from build123d import *

# Parameters (mm, degrees)
SKETCH1_R                  = 92.5
BOSS_EXTRUDE1_DEPTH        = 12
SKETCH2_OUTSIDE_W          = 239.38
SKETCH2_OUTSIDE_H          = 239.38
SKETCH2_OUTSIDE_W_2        = 140
SKETCH2_OUTSIDE_H_2        = 140
CUT_EXTRUDE1_DEPTH         = 132.363998112
SKETCH3_R                  = 65
CUT_EXTRUDE2_DEPTH         = 100.719606899
F_12_0_12_DIAMETER_HOLE1_D = 12


with BuildPart() as part:
    # Sketch1 → Boss-Extrude1 (new body)
    with BuildSketch(Plane.XY):
        Circle(SKETCH1_R)
    extrude(amount=BOSS_EXTRUDE1_DEPTH)

    # Sketch2 outside → Cut-Extrude1 (cut, through all)
    with BuildSketch(Plane.XY.offset(12)):
        Rectangle(SKETCH2_OUTSIDE_W, SKETCH2_OUTSIDE_H)
        Rectangle(SKETCH2_OUTSIDE_W_2, SKETCH2_OUTSIDE_H_2, mode=Mode.SUBTRACT)
    extrude(amount=-CUT_EXTRUDE1_DEPTH, mode=Mode.SUBTRACT)

    # Sketch3 → Cut-Extrude2 (cut, through all)
    with BuildSketch(Plane.XY.offset(12)):
        Circle(SKETCH3_R)
    extrude(amount=-CUT_EXTRUDE2_DEPTH, mode=Mode.SUBTRACT)

    # Ø12.0 (12) Diameter Hole1 (through all)
    with Locations(Plane.XY.offset(12)):
        with Locations((56.568542495, 56.568542495), (-56.568542495, 56.568542495), (-56.568542495, -56.568542495), (56.568542495, -56.568542495)):
            Hole(F_12_0_12_DIAMETER_HOLE1_D / 2)


solid = part.part
Part model, mm, in its own coordinate system. Give positions to 0.01 mm unless a question says otherwise; leave off trailing zeros. Loops run counter-clockwise (first coordinate to the right, second up) from the corner with the lowest first, then second, coordinate; pieces in that order, holes last.
(1) Band-saw the part on A-A (x = 39). Write the cut outline in (y, z), and give its area (3 significant figures).
Return value:
outline: (-70, 0) - (-52, 0) - (-52, 12) - (-70, 12) - close; (52, 0) - (70, 0) - (70, 12) - (52, 12) - close
area: 432 mm2
(2) Pull direction X, two halves, no side cores. Call faces 1 (the cylindrical face through (65.341, -65.474, 5.916)), 2 (the flat face through (-1, 70, 6)), 3 (the cylindrical face through (-62.11, 54.27, 5.92)), 4 (the flat face through (-70, -1, 6)): pulls with the +X half, pulls with the -X half, needs draft (parallel to the pull), parting line crosses it, or undercut.
Return value:
face 1: pulls with the +X half
face 2: needs draft
face 3: undercut
face 4: pulls with the -X half
(3) Band-saw the part on B-B (y = -16). Write the cut outline in (x, z).
Return value:
outline: (-70, 0) - (-63, 0) - (-63, 12) - (-70, 12) - close; (63, 0) - (70, 0) - (70, 12) - (63, 12) - close
(4) Drill centre lines: line 1 along Y through (x, z) = (2.5, 5); line 2 along Y through (x, z) = (16.5, 2.75); line 3 along Y through (x, z) = (-56.5, 6). Where is each one in solid material? Low to high.
Return value:
line 1: y = -70 to -64.95, 64.95 to 70
line 2: y = -70 to -62.87, 62.87 to 70
line 3: y = -70 to -62.57, -50.57 to -32.14, 32.14 to 50.57, 62.57 to 70
(5) Band-saw the part on C-C (z = 6). Write the cut outline in (x, y).
Return value:
outline: (-70, -60.47) arc R92.5 ccw to (-60.47, -70) - (60.47, -70) arc R92.5 ccw to (70, -60.47) - (70, 60.47) arc R92.5 ccw to (60.47, 70) - (-60.47, 70) arc R92.5 ccw to (-70, 60.47) - close; hole circle Ø130 at (0, 0); hole circle Ø12 at (-56.57, -56.57); hole circle Ø12 at (-56.57, 56.57); hole circle Ø12 at (56.57, -56.57); hole circle Ø12 at (56.57, 56.57)
